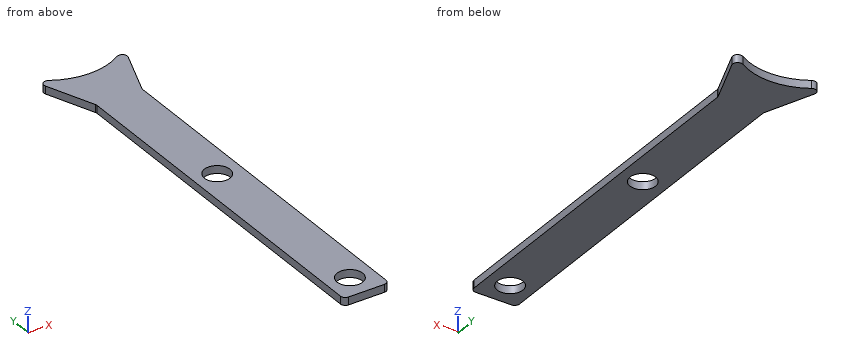
```python
from build123d import *

# Parameters (mm, degrees)
SKETCH1_R           = 2.625
BOSS_EXTRUDE1_DEPTH = 1.5875
FILLET1_R           = 1


with BuildPart() as part:
    # Sketch1 → Boss-Extrude1 (new body)
    with BuildSketch(Plane.XY):
        with BuildLine():
            Line((-11.271295364, 58.066064539), (-6.099639673, 44.56328746))
            Line((-6.099639673, 44.56328746), (-6.099639673, -30.902312688))
            Line((-6.099639673, -30.902312688), (3.214360327, -30.902312688))
            Line((3.214360327, -30.902312688), (3.214360327, 44.56328746))
            Line((3.214360327, 44.56328746), (8.386016017, 58.066064539))
            ThreePointArc((8.386016017, 58.066064539), (-1.442639673, 53.681260746), (-11.271295364, 58.066064539))
        make_face()
        with Locations((-1.442639673, 14.68417415)):
            Circle(SKETCH1_R, mode=Mode.SUBTRACT)
        with Locations((-1.442639673, -25.828822829)):
            Circle(SKETCH1_R, mode=Mode.SUBTRACT)
    extrude(amount=BOSS_EXTRUDE1_DEPTH)

    # Fillet1
    fillet1_edges = [part.edges().sort_by_distance(p)[0] for p in [
        (3.214360327, -30.902312688, 0.79375),
        (-6.099639673, -30.902312688, 0.79375),
        (-6.099639673, 44.56328746, 0.79375),
        (-11.271295364, 58.066064539, 0.79375),
        (8.386016017, 58.066064539, 0.79375),
        (3.214360327, 44.56328746, 0.79375),
    ]]
    fillet(fillet1_edges, radius=FILLET1_R)


solid = part.part
```
Can you work these out from the model? Positions are in its coordinate system, mm. Coordinates: 2 decimals unless noted, no trailing zeros. Order: outer loops, then holes, each group sorted by start corner. A loop starts at its lowest first (then second) coordinate and runs counter-clockwise, first axis right, second up. Notation, with made-up numbers: (-4.75, 80) -> (42.25, 80) arc R12 ccw to (42.25, 85) -> close; hole circle Ø11 at (-7, 42). An arc over 180 degrees is marked (long way). Write each question's results on one line, items separated by ' | '.
Item 1: I want a section at D-D, the plane y = 40. Write out the boundary of the cut face in (x, z).
Results are:
outline: (-6.1, 0) -> (3.21, 0) -> (3.21, 1.59) -> (-6.1, 1.59) -> close
Item 2: If I drill on line 1 along Y through (x, z) = (-0.25, 1.5); line 2 along X through (y, z) = (-17, 0.25); line 3 along Y through (x, z) = (-0.5, 1.5), over which ranges is the centre line in solid material (lowest first)?
Results are:
line 1: -30.9 to -28.17, -23.49 to 12.35, 17.02 to 53.74 | line 2: -6.1 to 3.21 | line 3: -30.9 to -28.28, -23.38 to 12.23, 17.13 to 53.71
Item 3: I want a section at A-A, the plane y = 16.5. Write out the boundary of the cut face in (x, z).
Results are:
outline: (-6.1, 0) -> (-3.34, 0) -> (-3.34, 1.59) -> (-6.1, 1.59) -> close; (0.45, 0) -> (3.21, 0) -> (3.21, 1.59) -> (0.45, 1.59) -> close
Item 4: I want a section at B-B, the plane x = -2. Write out the boundary of the cut face in (y, z).
Results are:
outline: (-30.9, 0) -> (-28.39, 0) -> (-28.39, 1.59) -> (-30.9, 1.59) -> close; (-23.26, 0) -> (12.12, 0) -> (12.12, 1.59) -> (-23.26, 1.59) -> close; (17.25, 0) -> (53.69, 0) -> (53.69, 1.59) -> (17.25, 1.59) -> close
Item 5: I'm going to push flat-ended pins straight in: pin 1 Ø6 at (x, y) = (0, -12.5) entering from -Z; pin 2 Ø4.5 at (x, y) = (-1.44, -25.83) entering from +Z; pin 3 Ø0.8 at (y, z) = (-6, 0.5) entering from -X. Where does each tip first touch, or does it pass through?
Results are:
pin 1: z = 0 | pin 2: through | pin 3: x = -6.1
Item 6: I want a section at C-C, the plane z = 0.95. Count the separate pieces of the cut face and the enclosed holes in it, then the cut area to 3 significant figures.
Results are:
separate pieces: 1 | enclosed holes: 2 | area: 791 mm²
